Design review of the part built by this model. Coordinates are the model's own, in mm. A direction names the side the tool comes from. Give positions to 0.01 mm unless a question says otherwise; leave off trailing zeros. Write each loop counter-clockwise with the first axis right and the second up, starting at its lowest first coordinate (ties: lowest second). Pieces come first, ordered by that corner, then holes. Notation, with made-up numbers: (10, -24.75) -> (64, -24.75) arc R26 ccw to (64, 11.25) -> close; hole circle Ø1 at (78, -11.5). An arc over 180 degrees is marked (long way). Write each question's results on one line, items separated by ' | '. Start each with the question number.
(1) For faces 1 (the face through (0.736, -1.972, -2.337)), 2 (the face through (-7.81, 1.08, -1.73)), list the 3-axis set-ups (+Z, -Z, +X, -X, +Y, -Y) from which the entire face can be reached by the end or side of a thin tool; tool diameter is ignored.
(2) Take a section at B-B (x = 0). State the section outline as (y, z) points, plus the area to 3 significant figures.
(3) Clearance check with a flat-ended pin moving along its axis: pin 1 (4.5 mm diameter, centred on x = 0, z = 0, fed in from -Y). State where the tip first meets the part, or that it passes through.
(4) Take a section at D-D (z = -2.75). State the section outline as (x, y) points, plus the area to 3 significant figures.
(5) Mouldability with a two-part tool opening along X and no side actions: class faces 3 (the face through (-0.9, -1.97, 2.86)), 4 (the face through (-2, 2.2, 0)), 5 (the face through (0.39, 1.12, -3.26)) as released by +X, released by -X, zero draft, split by the parting line, or undercut.
(6) Take a section at C-C (y = 0.25). State the section outline as (x, z) points, plus the area to 3 significant figures.
(7) To check wall thickness, follow probe 1 along X at (y, z) = (1.7, 0); probe 2 along X at (y, z) = (-1.25, 0); probe 3 along Y at (x, z) = (0.25, -6.5). State the ranges of each line that lie inside material, in increasing order.
(8) Take a section at A-A (z = 0). State the section outline as (x, y) points, plus the area to 3 significant figures.
from build123d import *

# Parameters (mm, degrees)
SKETCH1_R           = 8
BOSS_EXTRUDE1_DEPTH = 2.2
SKETCH2_R           = 1.3
CUT_EXTRUDE1_DEPTH  = 2.2
SKETCH3_R           = 3
SKETCH3_R_2         = 2.45
BOSS_EXTRUDE2_DEPTH = 4
SKETCH8_R           = 0.6
CUT_EXTRUDE7_DEPTH  = 2.2


with BuildPart() as part:
    # Sketch1 → Boss-Extrude1 (new body)
    with BuildSketch(Plane(origin=(0, 0, 0), x_dir=(1, 0, 0), z_dir=(0, 1, 0))):
        with Locations(Location((0, 0, 0), (0, 0, 270))):
            Circle(SKETCH1_R)
    extrude(amount=BOSS_EXTRUDE1_DEPTH)

    # Sketch2 → Cut-Extrude1 (cut)
    with BuildSketch(Plane(origin=(0, 2.2, 0), x_dir=(1, 0, 0), z_dir=(0, 1, 0))):
        with Locations(Location((0, 4.5, 0), (0, 0, 270))):
            Circle(SKETCH2_R)
        with Locations(Location((0, -4.5, 0), (0, 0, 90))):
            Circle(SKETCH2_R)
    extrude(amount=-CUT_EXTRUDE1_DEPTH, mode=Mode.SUBTRACT)

    # Sketch3 → Boss-Extrude2 (add)
    with BuildSketch(Plane.XZ):
        with Locations(Location((0, 0, 0), (0, 0, 90))):
            Circle(SKETCH3_R)
        with Locations(Location((0, 0, 0), (0, 0, 270))):
            Circle(SKETCH3_R_2, mode=Mode.SUBTRACT)
    extrude(amount=BOSS_EXTRUDE2_DEPTH)

    # Sketch8 → Cut-Extrude7 (cut)
    with BuildSketch(Plane.XZ):
        with Locations(Location((0, 0, 0), (0, 0, 270))):
            Circle(SKETCH8_R)
    extrude(amount=-CUT_EXTRUDE7_DEPTH, mode=Mode.SUBTRACT)


solid = part.part
Report:
1) face 1: -Y | face 2: +Y, -Y
2) outline: (-4, -3) -> (0, -3) -> (0, -3.2) -> (2.2, -3.2) -> (2.2, -0.6) -> (0, -0.6) -> (0, -2.45) -> (-4, -2.45) -> close; (-4, 2.45) -> (0, 2.45) -> (0, 0.6) -> (2.2, 0.6) -> (2.2, 3.2) -> (0, 3.2) -> (0, 3) -> (-4, 3) -> close; (0, -8) -> (2.2, -8) -> (2.2, -5.8) -> (0, -5.8) -> close; (0, 5.8) -> (2.2, 5.8) -> (2.2, 8) -> (0, 8) -> close | area: 25.5 mm2
3) pin 1: y = 0
4) outline: (-7.51, 0) -> (-1.2, 0) -> (-1.2, -4) -> (1.2, -4) -> (1.2, 0) -> (7.51, 0) -> (7.51, 2.2) -> (-7.51, 2.2) -> close | area: 42.6 mm2
5) face 3: split by the parting line | face 4: zero draft | face 5: undercut
6) outline: circle Ø16 at (0, 0); hole circle Ø2.6 at (0, -4.5); hole circle Ø2.6 at (0, 4.5); hole circle Ø1.2 at (0, 0) | area: 189 mm2
7) probe 1: -8 to -0.6, 0.6 to 8 | probe 2: -3 to -2.45, 2.45 to 3 | probe 3: 0 to 2.2
8) outline: (-8, 0) -> (-3, 0) -> (-3, -4) -> (-2.45, -4) -> (-2.45, 0) -> (-0.6, 0) -> (-0.6, 2.2) -> (-8, 2.2) -> close; (0.6, 0) -> (2.45, 0) -> (2.45, -4) -> (3, -4) -> (3, 0) -> (8, 0) -> (8, 2.2) -> (0.6, 2.2) -> close | area: 37.0 mm2
